Could you check a few things on this model? Use its own coordinates, in mm. Face numbers are marked on the shaded views. Round coordinates to 2 decimals unless told otherwise and drop trailing zeros. Write each loop counter-clockwise with the first axis right and the second up, starting at its lowest first coordinate (ties: lowest second). Pieces come first, ordered by that corner, then holes. Notation, with made-up numbers: (-24, -6) - (-16, -6) arc R24 ccw to (-16, 18) - close; hole circle Ø5 at (58, 50). An arc over 180 degrees is marked (long way). Put each result on its own line as item: value.
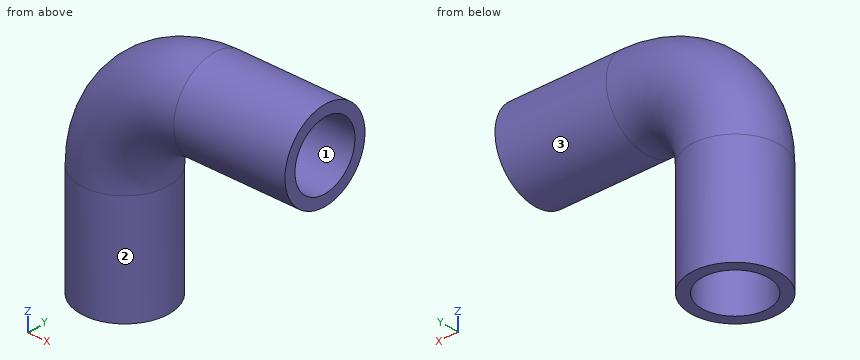
from build123d import *

# Parameters (mm, degrees)
F0_R     = 10
F0_R_2   = 7.5
F1_DEPTH = 25
F3_R     = 10
F3_R_2   = 7.5
F4_ANGLE = 90
F5_DEPTH = 25


with BuildPart() as f1:
    # F0 (on Top) → F1 (new body)
    with BuildSketch(Plane.XY):
        Circle(F0_R)
        Circle(F0_R_2, mode=Mode.SUBTRACT)
    extrude(amount=F1_DEPTH)

    # F3 (on face) → F4 (revolve)
    with BuildSketch(Plane.XY.offset(25)):
        Circle(F3_R)
        Circle(F3_R_2, mode=Mode.SUBTRACT)
    revolve(axis=Axis((20, 0.0099948445, 25), (0, 1, 0)), revolution_arc=F4_ANGLE)

    # F5 (add): a face of the model
    f5_faces = [f1.faces().sort_by_distance(p)[0] for p in [
        (20, 0, 54.7171572875),
    ]]
    extrude(f5_faces, amount=F5_DEPTH)


solid = f1.part
(1) Imagine slicing it at B-B, the plane y = 8.75. List the corners of the cut face in (x, z) for me, then the cut area to 3 significant figures.
Values found:
outline: (-4.84, 0) - (4.84, 0) - (4.84, 25) arc R15.16 cw to (20, 40.16) - (45, 40.16) - (45, 49.84) - (20, 49.84) arc R24.84 ccw to (-4.84, 25) - close
area: 788 mm^2
(2) If we mould it in two halves opening along Z, with no side actions, what happens to the marked faces 1, 2 and 3? For each: pulls with the +Z half, pulls with the -Z half, needs draft (parallel to the pull), parting line crosses it, or undercut.
Values found:
face 1: undercut
face 2: needs draft
face 3: parting line crosses it
(3) I'm going to push flat-ended pins straight in: pin 1 (1.5 mm diameter, centred on x = -2, y = 2, fed in from -Z); pin 2 (12 mm diameter, centred on x = 39.5, z = 31, fed in from +Y); pin 3 (4 mm diameter, centred on y = 4, z = 8.5, fed in from -X). Where does each tip first touch, or does it pass through?
Values found:
pin 1: stops at z = 39.89
pin 2: stops at y = 6
pin 3: stops at x = -9.8
(4) Imagine slicing it at D-D, the plane x = 23.5. List the corners of the cut face in (y, z) for me.
Values found:
outline: circle Ø20 at (0, 45); hole circle Ø15 at (0, 45)
(5) Imagine slicing it at A-A, the plane y = 0. List the corners of the cut face in (x, z) for me.
Values found:
outline: (-10, 0) - (-7.5, 0) - (-7.5, 25) arc R27.5 cw to (20, 52.5) - (45, 52.5) - (45, 55) - (20, 55) arc R30 ccw to (-10, 25) - close; (7.5, 0) - (10, 0) - (10, 25) arc R10 cw to (20, 35) - (45, 35) - (45, 37.5) - (20, 37.5) arc R12.5 ccw to (7.5, 25) - close
(6) Please list where these lines run through material, in increasing order: probe 1 along Y at (x, z) = (0, 12.5); probe 2 along Z at (x, y) = (28, 3); probe 3 along Y at (x, z) = (-5.5, 24.5). Write a range as from..to.
Values found:
probe 1: y = -10..-7.5, 7.5..10
probe 2: z = 35.46..38.13, 51.87..54.54
probe 3: y = -8.35..-5.1, 5.1..8.35
(7) Imagine slicing it at C-C, the plane z = 13. List the corners of the cut face in (x, y) for me, then the cut area to 3 significant figures.
Values found:
outline: circle Ø20 at (0, 0); hole circle Ø15 at (0, 0)
area: 137 mm^2
